from build123d import *

# Parameters (mm, degrees)
F0_W     = 89
F0_H     = 89
F1_DEPTH = 40
F2_R     = 30
F3_DEPTH = 50


with BuildPart() as f1:
    # F0 (on Top) → F1 (new body)
    with BuildSketch(Plane.XY):
        Rectangle(F0_W, F0_H)
    extrude(amount=F1_DEPTH)

    # F2 (on face) → F3 (join)
    with BuildSketch(Plane(origin=(0, 0, 0), x_dir=(1, 0, 0), z_dir=(0, 0, -1))):
        Circle(F2_R)
    extrude(amount=F3_DEPTH)


solid = f1.part
For this review, take the finished solid that the model builds, in its own axes (mm). A direction names the side the tool comes from. Coordinates: 2 decimals unless noted, no trailing zeros. Order: outer loops, then holes, each group sorted by start corner. A loop starts at its lowest first (then second) coordinate and runs counter-clockwise, first axis right, second up. Notation, with made-up numbers: (19, 11) -> (74, 11) arc R33 cw to (74, 50) -> close; hole circle Ø1 at (-19.5, 37). An arc over 180 degrees is marked (long way). Return JSON: item names as keys, results as strings.
1. We need section C-C on z = -7. Write out the cut boundary in (x, y), and give its area (3 significant figures).
Answer block:
{"outline": "circle Ø60 at (0, 0)", "area": "2,830 mm²"}
2. We need section A-A on y = 0. Write out the cut boundary in (x, z), and give its area (3 significant figures).
Answer block:
{"outline": "(-44.5, 0) -> (-30, 0) -> (-30, -50) -> (30, -50) -> (30, 0) -> (44.5, 0) -> (44.5, 40) -> (-44.5, 40) -> close", "area": "6,560 mm²"}
3. We need section D-D on x = -35. Write out the cut boundary in (y, z), and give its area (3 significant figures).
Answer block:
{"outline": "(-44.5, 0) -> (44.5, 0) -> (44.5, 40) -> (-44.5, 40) -> close", "area": "3,560 mm²"}
4. For line 1 (Z direction, x = 31, y = -1.5); line 2 (X direction, y = -6.5, z = -43); line 3 (Y direction, x = 11, z = -9.5), list the stretches that pass through material, from the lowest coordinate up. Write a range as from..to.
Answer block:
{"line 1": "0..40", "line 2": "-29.29..29.29", "line 3": "-27.91..27.91"}
5. For pin 1 Ø2 at (x, z) = (2.5, -13) entering from +Y, flat-tipped, find the tip position at first contact; note if it passes through.
Answer block:
{"pin 1": "y = 29.96"}
6. We need section B-B on x = -11. Write out the cut boundary in (y, z), and give its area (3 significant figures).
Answer block:
{"outline": "(-44.5, 0) -> (-27.91, 0) -> (-27.91, -50) -> (27.91, -50) -> (27.91, 0) -> (44.5, 0) -> (44.5, 40) -> (-44.5, 40) -> close", "area": "6,350 mm²"}
7. Machinability: for faces 1 (the cylindrical face through (-29.97, -1.32, -24.65)), 2 (the flat face through (0, 0, -50)), which of the approach directions +Z, -Z, +X, -X, +Y, -Y give a long, thin tool a straight path to every point of the face, cutting with its end or side? Answer none if there is none.
Answer block:
{"face 1": "-Z", "face 2": "-Z, +X, -X, +Y, -Y"}
